```python
from build123d import *

# Parameters (mm, degrees)
ESTRUSIONE_ESTRUSIONE1_DEPTH  = 5
FORO_FILETTATO_M3X0_5_1_D     = 2.5
FORO_FILETTATO_M3X0_5_1_DEPTH = 7.5
FORO_FILETTATO_M3X0_5_1_TIP   = 0.751075774
SCHIZZO4_W                    = 69.084596206
SCHIZZO4_H                    = 3
TAGLIO_ESTRUSIONE2_DEPTH      = 10
SCHIZZO7_W                    = 3
SCHIZZO7_H                    = 47.5
TAGLIO_ESTRUSIONE5_DEPTH      = 10
SCHIZZO12_W                   = 3
SCHIZZO12_H                   = 40
TAGLIO_ESTRUSIONE8_DEPTH      = 237.814801058
TAGLIO_ESTRUSIONE1_DEPTH      = 237.814801058
TAGLIO_ESTRUSIONE1_DEPTH_BACK = 237.814801058
FORO_FILETTATO_M3X0_5_4_D     = 2.5
RACCORDO1_R                   = 8
RACCORDO2_R                   = 10


with BuildPart() as part:
    # Schizzo1 → Estrusione-Estrusione1 (new body)
    with BuildSketch(Plane(origin=(0, 0, 0), x_dir=(1, 0, 0), z_dir=(0, 1, 0))):
        Polygon((65, 67.5), (65, 87.5), (160.052105959, 87.5), (201.585225273, 70.801270189), (220, 30), (220, -30), (201.585225273, -70.801270189), (160.052105959, -87.5), (65, -87.5), (65, -67.5), (0, -67.5), (0, 67.5), align=None)
    extrude(amount=ESTRUSIONE_ESTRUSIONE1_DEPTH)

    # Foro filettato M3x0.5-1
    with Locations(Plane(origin=(0, 5, 0), x_dir=(1, 0, 0), z_dir=(0, 1, 0))):
        with Locations((197.854862265, 66.912097904), (215, 28.92393853), (215, -28.92393853), (197.854862265, -66.912097904), (159.084596206, -82.5), (159.084596206, 82.5), (70, 82.5), (70, -82.5), (5, -62.5), (5, 62.5)):
            Hole(FORO_FILETTATO_M3X0_5_1_D / 2, depth=FORO_FILETTATO_M3X0_5_1_DEPTH)
            with Locations((0, 0, -(FORO_FILETTATO_M3X0_5_1_DEPTH + FORO_FILETTATO_M3X0_5_1_TIP / 2))):  # 118° drill point
                Cone(0, FORO_FILETTATO_M3X0_5_1_D / 2, FORO_FILETTATO_M3X0_5_1_TIP, mode=Mode.SUBTRACT)

    # Schizzo4 → Taglio-Estrusione2 (cut)
    with BuildSketch(Plane(origin=(0, 5, 0), x_dir=(1, 0, 0), z_dir=(0, 1, 0))):
        with Locations((114.542298103, -82.5)):
            Rectangle(SCHIZZO4_W, SCHIZZO4_H)
        Polygon((209.519084515, 37.421559693), (200.601374282, 57.180362615), (203.33577775, 58.414476741), (212.253487983, 38.655673819), align=None)
        with Locations((114.542298103, 82.5)):
            Rectangle(SCHIZZO4_W, SCHIZZO4_H)
        Polygon((189.136249234, 72.034186035), (168.92231814, 80.161362114), (167.803209237, 77.377911869), (188.017140331, 69.250735791), align=None)
        Polygon((167.803209237, -77.377911869), (188.017140331, -69.250735791), (189.136249234, -72.034186035), (168.92231814, -80.161362114), align=None)
        Polygon((200.601374282, -57.180362615), (209.519084515, -37.421559693), (212.253487983, -38.655673819), (203.33577775, -58.414476741), align=None)
    extrude(amount=-TAGLIO_ESTRUSIONE2_DEPTH, mode=Mode.SUBTRACT)

    # Schizzo7 → Taglio-Estrusione5 (cut)
    with BuildSketch(Plane(origin=(0, 5, 0), x_dir=(1, 0, 0), z_dir=(0, 1, 0))):
        with Locations((5, 28.75)):
            Rectangle(SCHIZZO7_W, SCHIZZO7_H)
        with Locations((5, -28.75)):
            Rectangle(SCHIZZO7_W, SCHIZZO7_H)
    extrude(amount=-TAGLIO_ESTRUSIONE5_DEPTH, mode=Mode.SUBTRACT)

    # Schizzo12 → Taglio-Estrusione8 (cut, through all)
    with BuildSketch(Plane(origin=(0, 5, 0), x_dir=(1, 0, 0), z_dir=(0, 1, 0))):
        with Locations((72.042298103, 0)):
            Rectangle(SCHIZZO12_W, SCHIZZO12_H)
    extrude(amount=-TAGLIO_ESTRUSIONE8_DEPTH, mode=Mode.SUBTRACT)

    # Schizzo2 → Taglio-Estrusione1 (cut, two sides: drawn at the far end of the back side and taken through both)
    with BuildSketch(Plane(origin=(0, 5, 0), x_dir=(1, 0, 0), z_dir=(0, 1, 0)).offset(-TAGLIO_ESTRUSIONE1_DEPTH_BACK)):
        Polygon((719.281105296, 19.5), (220, 19.5), (190, 19.5), (190, -19.5), (220, -19.5), (719.281105296, -19.5), (1717.843315889, -19.5), (1717.843315889, 19.5), align=None)
    extrude(amount=TAGLIO_ESTRUSIONE1_DEPTH + TAGLIO_ESTRUSIONE1_DEPTH_BACK, mode=Mode.SUBTRACT)

    # Foro filettato M3x0.5-4 (through all)
    with Locations(Plane(origin=(0, 5, 0), x_dir=(1, 0, 0), z_dir=(0, 1, 0))):
        with Locations((189, 26.5), (189, -26.5)):
            Hole(FORO_FILETTATO_M3X0_5_4_D / 2)

    # Raccordo1
    raccordo1_edges = [part.edges().sort_by_distance(p)[0] for p in [
        (0, 2.5, -67.5),
        (65, 2.5, -67.5),
        (65, 2.5, -87.5),
        (65, 2.5, 87.5),
        (65, 2.5, 67.5),
        (0, 2.5, 67.5),
    ]]
    fillet(raccordo1_edges, radius=RACCORDO1_R)

    # Raccordo2
    raccordo2_edges = [part.edges().sort_by_distance(p)[0] for p in [
        (160.052105959, 2.5, -87.5),
        (201.585225273, 2.5, -70.801270189),
        (220, 2.5, -30),
        (220, 2.5, 30),
        (201.585225273, 2.5, 70.801270189),
        (160.052105959, 2.5, 87.5),
    ]]
    fillet(raccordo2_edges, radius=RACCORDO2_R)


solid = part.part
```
The model under review builds one solid part; all positions refer to its coordinate system, in mm. A direction names the side the tool comes from. Coordinates: 2 decimals unless noted, no trailing zeros. Write each loop counter-clockwise with the first axis right and the second up, starting at its lowest first coordinate (ties: lowest second). Pieces come first, ordered by that corner, then holes.
1) We need section A-A on x = 131.5. State the section outline as (y, z) points.
2) The part is to be moulded in two halves that separate along Z. For faces 1 (the face through (201.008, 2.535, -70.277)), 2 (the face through (220, 2, -24)), 3 (the face through (205, 2, -19.5)), 4 (the face through (180.1, 2.46, 79.44)), say which applies: pulls with the +Z half, pulls with the -Z half, needs draft (parallel to the pull), parting line crosses it, or undercut.
3) We need section B-B on z = 42. State the section outline as (x, y) points.
4) Clearance check with flat-ended pins moving along their axes: pin 1 Ø2 at (x, z) = (215, -28.92) entering from +Y; pin 2 Ø0.9 at (x, y) = (71.5, 3.5) entering from +Z; pin 3 Ø2.5 at (x, y) = (44, 3.5) entering from -Z; pin 4 Ø0.9 at (x, y) = (4.5, 3) entering from +Z. State where each tip first meets the part, or that it passes through.
5) Machinability: for faces 5 (the face through (205, 2, 19.5)), 6 (the face through (62.719, 2.535, -69.906)), 7 (the face through (3.5, 3, 29)), which of the approach directions +Z, -Z, +X, -X, +Y, -Y give a long, thin tool a straight path to every point of the face, cutting with its end or side? Answer none if there is none.
6) We need section C-C on y = 1.8. Count the separate pieces of the cut face and the enclosed holes in it, then the cut area to 3 significant figures.
7) To check wall thickness, follow probe 1 along X at (y, z) = (3.15, 26.5); probe 2 along Z at (x, y) = (123.5, 1.65); probe 3 along X at (y, z) = (3.35, 18). State the ranges of each line that lie inside material, in increasing order.
Answer list:
1. outline: (0, -87.5) - (5, -87.5) - (5, -84) - (0, -84) - close; (0, -81) - (5, -81) - (5, 81) - (0, 81) - close; (0, 84) - (5, 84) - (5, 87.5) - (0, 87.5) - close
2. face 1: pulls with the -Z half
2. face 2: needs draft
2. face 3: undercut
2. face 4: pulls with the +Z half
3. outline: (0, 0) - (3.5, 0) - (3.5, 5) - (0, 5) - close; (6.5, 0) - (207.45, 0) - (207.45, 5) - (6.5, 5) - close; (210.74, 0) - (214.58, 0) - (214.58, 5) - (210.74, 5) - close
4. pin 1: passes through
4. pin 2: stops at z = 87.43
4. pin 3: stops at z = -67.5
4. pin 4: stops at z = 66.9
5. face 5: +X, +Y, -Y
5. face 6: -Z, -X, +Y, -Y
5. face 7: +Y, -Y
6. separate pieces: 1
6. enclosed holes: 21
6. area: 31,500 mm2
7. probe 1: x = 0 to 3.5, 6.5 to 187.75, 190.25 to 220
7. probe 2: z = -87.5 to -84, -81 to 81, 84 to 87.5
7. probe 3: x = 0 to 3.5, 6.5 to 70.54, 73.54 to 190
